Source: CAD feature listing. Evaluate the final solid. Frame: model axes, mm. Face numbers are marked on the shaded views. A direction names the side the tool comes from. Give positions to 0.01 mm unless a question says otherwise; leave off trailing zeros. Order: outer loops, then holes, each group sorted by start corner. A loop starts at its lowest first (then second) coordinate and runs counter-clockwise, first axis right, second up.
1) Section A-A, the plane x = 43. Return loops of the section in (y, z), plus the area to 3 significant figures.
2) Section D-D, the plane x = 60. Return loops of the section in (y, z).
3) Section C-C, the plane z = -6. Return loops of the section in (x, y), plus the area to 3 significant figures.
4) Access query for the marked faces 1 and 2. Directions: +Z, -Z, +X, -X, +Y, -Y. A direction counts if a zero-diameter tool reaches every point of the face in a straight line with its end or side. Return the directions, or none.
5) Material intervals for line 1 (X direction, y = 1.3, z = -12.5); line 2 (Y direction, x = 17, z = -10.5); line 3 (X direction, y = 55.35, z = -12.5), sorted ascending.
6) Section B-B, the plane y = 34.15. Return loops of the section in (x, z), plus the area to 3 significant figures.
7) First-contact query: P1, Ø2.5, axis at x = 19, z = -12.5, coming from the +Y side; P2, Ø5, axis at y = 12.5, z = -13.5, coming from the +X side. Flat tips, straight axial feed; report the tip coordinate or a pass-through.
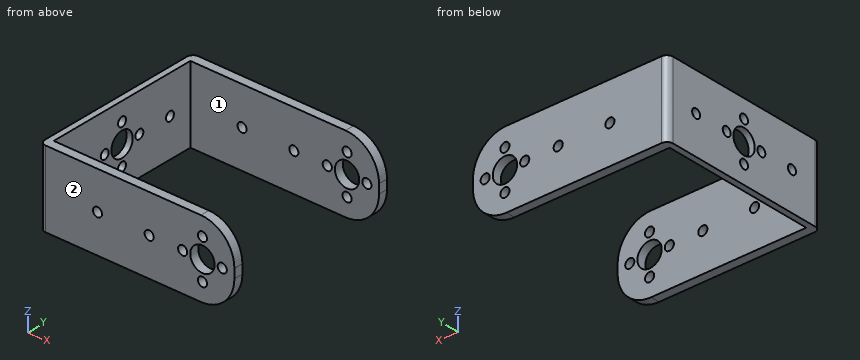
```python
from build123d import *

# Parameters (mm, degrees)
BOSS_EXTRUDE1_DEPTH      = 56.3
BOSS_EXTRUDE1_DEPTH_BACK = 1
SKETCH1_W                = 64
SKETCH1_H                = 25
SKETCH3_W                = 62
SKETCH3_H                = 51.3
CUT_EXTRUDE2_DEPTH       = 89.829555892
SKETCH4_R                = 4
SKETCH4_R_2              = 1.5
CUT_EXTRUDE3_DEPTH       = 56
SKETCH8_R                = 1.5
CUT_EXTRUDE4_DEPTH       = 56
FILLET1_R                = 2
SKETCH9_R                = 1.5
SKETCH9_R_2              = 4
CUT_EXTRUDE5_DEPTH       = 90.466697715
FILLET3_R                = 11
SKETCH10_R               = 1.5
CUT_EXTRUDE6_DEPTH       = 90.466697715


with BuildPart() as part:
    # Sketch1 → Boss-Extrude1 (new, two sides: drawn at the far end of the back side and taken through both)
    with BuildSketch(Plane(origin=(0, 0, 0), x_dir=(1, 0, 0), z_dir=(0, 1, 0)).offset(-BOSS_EXTRUDE1_DEPTH_BACK)):
        with Locations((32, 12.5)):
            Rectangle(SKETCH1_W, SKETCH1_H)
    extrude(amount=BOSS_EXTRUDE1_DEPTH + BOSS_EXTRUDE1_DEPTH_BACK)

    # Sketch3 → Cut-Extrude2 (cut, through all)
    with BuildSketch(Plane.XY):
        with Locations((33, 27.65)):
            Rectangle(SKETCH3_W, SKETCH3_H)
    extrude(amount=-CUT_EXTRUDE2_DEPTH, mode=Mode.SUBTRACT)

    # Sketch4 → Cut-Extrude3 (cut)
    with BuildSketch(Plane(origin=(2, 0, 0), x_dir=(0, 0, -1), z_dir=(1, 0, 0))):
        with Locations(Location((12.5, 27.65, 0), (0, 0, 90))):
            Circle(SKETCH4_R)
        with Locations(Location((19, 27.65, 0), (0, 0, 90))):
            Circle(SKETCH4_R_2)
        with Locations(Location((12.5, 34.15, 0), (0, 0, 90))):
            Circle(SKETCH4_R_2)
        with Locations(Location((6, 27.65, 0), (0, 0, 180))):
            Circle(SKETCH4_R_2)
        with Locations(Location((12.5, 21.15, 0), (0, 0, 180))):
            Circle(SKETCH4_R_2)
    extrude(amount=-CUT_EXTRUDE3_DEPTH, mode=Mode.SUBTRACT)

    # Sketch8 → Cut-Extrude4 (cut)
    with BuildSketch(Plane(origin=(2, 0, 0), x_dir=(0, 0, -1), z_dir=(1, 0, 0))):
        with Locations(Location((12.5, 45.65, 0), (0, 0, 90))):
            Circle(SKETCH8_R)
        with Locations(Location((12.5, 9.65, 0), (0, 0, 90))):
            Circle(SKETCH8_R)
    extrude(amount=-CUT_EXTRUDE4_DEPTH, mode=Mode.SUBTRACT)

    # Fillet1
    fillet1_edges = [part.edges().sort_by_distance(p)[0] for p in [
        (0, 56.3, -12.5),
        (0, -1, -12.5),
    ]]
    fillet(fillet1_edges, radius=FILLET1_R)

    # Sketch9 → Cut-Extrude5 (cut, through all)
    with BuildSketch(Plane(origin=(0, 56.3, 0), x_dir=(1, 0, 0), z_dir=(0, 1, 0))):
        with Locations(Location((60, 12.5, 0), (0, 0, 270))):
            Circle(SKETCH9_R)
        with Locations(Location((53.5, 12.5, 0), (0, 0, 270))):
            Circle(SKETCH9_R_2)
        with Locations(Location((53.5, 19, 0), (0, 0, 270))):
            Circle(SKETCH9_R)
        with Locations(Location((47, 12.5, 0), (0, 0, 270))):
            Circle(SKETCH9_R)
        with Locations(Location((53.5, 6, 0), (0, 0, 270))):
            Circle(SKETCH9_R)
    extrude(amount=-CUT_EXTRUDE5_DEPTH, mode=Mode.SUBTRACT)

    # Fillet3
    fillet3_edges = [part.edges().sort_by_distance(p)[0] for p in [
        (64, 54.8, 0),
        (64, 54.8, -25),
        (64, 0.5, -25),
        (64, 0.5, 0),
    ]]
    fillet(fillet3_edges, radius=FILLET3_R)

    # Sketch10 → Cut-Extrude6 (cut, through all)
    with BuildSketch(Plane(origin=(0, 56.3, 0), x_dir=(1, 0, 0), z_dir=(0, 1, 0))):
        with Locations(Location((36, 12.5, 0), (0, 0, 270))):
            Circle(SKETCH10_R)
        with Locations(Location((19, 12.5, 0), (0, 0, 270))):
            Circle(SKETCH10_R)
    extrude(amount=-CUT_EXTRUDE6_DEPTH, mode=Mode.SUBTRACT)


solid = part.part
```
From the geometry:
1. outline: (-1, -25) - (2, -25) - (2, 0) - (-1, 0) - close; (53.3, -25) - (56.3, -25) - (56.3, 0) - (53.3, 0) - close
1. area: 150 mm2
2. outline: (-1, -22.49) - (2, -22.49) - (2, -14) - (-1, -14) - close; (-1, -11) - (2, -11) - (2, -2.51) - (-1, -2.51) - close; (53.3, -22.49) - (56.3, -22.49) - (56.3, -14) - (53.3, -14) - close; (53.3, -11) - (56.3, -11) - (56.3, -2.51) - (53.3, -2.51) - close
3. outline: (0, 1) arc R2 ccw to (2, -1) - (52, -1) - (52, 2) - (2, 2) - (2, 26.15) - (0, 26.15) - close; (0, 29.15) - (2, 29.15) - (2, 53.3) - (52, 53.3) - (52, 56.3) - (2, 56.3) arc R2 ccw to (0, 54.3) - close; (55, -1) - (62.8, -1) - (62.8, 2) - (55, 2) - close; (55, 53.3) - (62.8, 53.3) - (62.8, 56.3) - (55, 56.3) - close
3. area: 454 mm2
4. face 1: +Z, -Z, +X
4. face 2: +Z, -Z, +X, -X, -Y
5. line 1: x = 0 to 17.5, 20.5 to 34.5, 37.5 to 45.5, 48.5 to 49.5, 57.5 to 58.5, 61.5 to 64
5. line 2: y = -1 to 2, 53.3 to 56.3
5. line 3: x = 0.3 to 17.5, 20.5 to 34.5, 37.5 to 45.5, 48.5 to 49.5, 57.5 to 58.5, 61.5 to 64
6. outline: (0, -25) - (2, -25) - (2, -14) - (0, -14) - close; (0, -11) - (2, -11) - (2, 0) - (0, 0) - close
6. area: 44.0 mm2
7. P1: passes through
7. P2: stops at x = 2
